Read the model definition and answer for the solid it produces. Units are mm, in the model's axes. Face numbers are marked on the shaded views. A direction names the side the tool comes from. Coordinates: 2 decimals unless noted, no trailing zeros. Write each loop counter-clockwise with the first axis right and the second up, starting at its lowest first coordinate (ties: lowest second). Pieces come first, ordered by that corner, then holes. Notation, with made-up numbers: (-12.5, -6) -> (22.5, -6) arc R17 ccw to (22.5, 20) -> close; hole circle Ø4 at (-33.75, 73.25). An arc over 180 degrees is marked (long way). One line per item, written item: value. Start each with the question number.
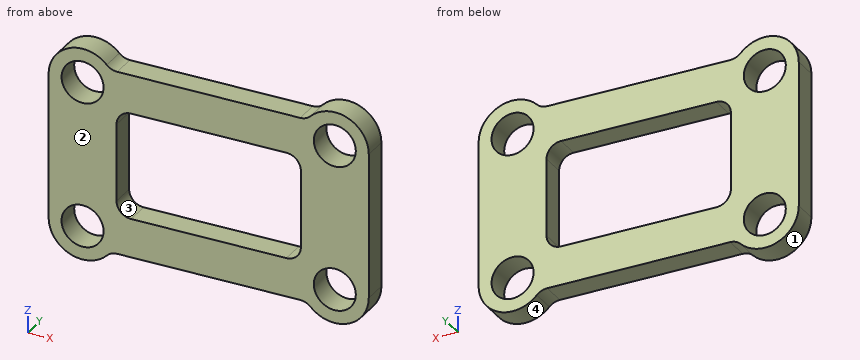
from build123d import *

# Parameters (mm, degrees)
BOSS_EXTRUDE2_DEPTH   = 3.175
BOSS_EXTRUDE2_2_DEPTH = 3.175
SKETCH7_W             = 33.02
SKETCH7_H             = 5.08
EXTRUDE_THIN1_DEPTH   = 3.175
M5_CLEARANCE_HOLE1_D  = 5.5
FILLET1_R             = 1.905


with BuildPart() as part:
    # Sketch1 → Boss-Extrude2 (new body)
    with BuildSketch(Plane.XZ.offset(19.05)):
        with BuildLine():
            Line((-24.765, 9.525), (-24.765, -9.525))
            ThreePointArc((-24.765, -9.525), (-29.21, -13.97), (-33.655, -9.525))
            Line((-33.655, -9.525), (-33.655, 9.525))
            ThreePointArc((-33.655, 9.525), (-29.21, 13.97), (-24.765, 9.525))
        make_face()
    extrude(amount=BOSS_EXTRUDE2_DEPTH)



with BuildPart() as body_2:
    # Sketch1 → Boss-Extrude2 2 (new body)
    with BuildSketch(Plane.XZ.offset(19.05)):
        with BuildLine():
            Line((8.255, 9.525), (8.255, -9.525))
            ThreePointArc((8.255, -9.525), (3.81, -13.97), (-0.635, -9.525))
            Line((-0.635, -9.525), (-0.635, 9.525))
            ThreePointArc((-0.635, 9.525), (3.81, 13.97), (8.255, 9.525))
        make_face()
    extrude(amount=BOSS_EXTRUDE2_2_DEPTH)


with BuildPart() as part_1:
    add(part.part)

    add(body_2.part)  # Extrude-Thin1 merges body 2
    # Sketch7 → Extrude-Thin1 (add)
    with BuildSketch(Plane.XZ.offset(22.225)):
        with Locations((-12.7, 9.525)):
            Rectangle(SKETCH7_W, SKETCH7_H)
        with Locations((-12.7, -9.525)):
            Rectangle(SKETCH7_W, SKETCH7_H)
    extrude(amount=-EXTRUDE_THIN1_DEPTH)

    # M5 Clearance Hole1 (through all)
    with Locations(Plane(origin=(-29.21, -22.225, 9.525), x_dir=(0, 0, -1), z_dir=(0, -1, 0))):
        with Locations((0, 0), (19.05, 0), (0, 33.02), (19.05, 33.02)):
            Hole(M5_CLEARANCE_HOLE1_D / 2)

    # Fillet1
    fillet1_edges = [part_1.edges().sort_by_distance(p)[0] for p in [
        (-25.562202719, -20.6375, 12.065),
        (-24.765, -20.6375, 6.985),
        (-0.635, -20.6375, 6.985),
        (0.162202719, -20.6375, 12.065),
        (0.162202719, -20.6375, -12.065),
        (-0.635, -20.6375, -6.985),
        (-24.765, -20.6375, -6.985),
        (-25.562202719, -20.6375, -12.065),
    ]]
    fillet(fillet1_edges, radius=FILLET1_R)


solid = part_1.part
1. A cutting plane is placed at D-D on x = -3. Give the vertices of the cut face in (y, z) (3 decimals).
2. A cutting plane is placed at A-A on y = -20.95. Count the separate pieces of the cut face and the enclosed holes in it, then the cut area to 3 significant figures.
3. A cutting plane is placed at C-C on z = -0.5. Give the vertices of the cut face in (x, y) (3 decimals).
4. Find the intervals of material crossed by probe 1 along Z at (x, y) = (-2.5, -20.95) (3 decimals); probe 2 along X at (y, z) = (-20.35, -8) (3 decimals); probe 3 along X at (y, z) = (-20.05, -11.75), in increasing order. Write a range as from..to.
5. A tool of negligible diameter and unlimited length cuts with its end or side. For the marked faces 3 and 4, from which of +Z, -Z, +X, -X, +Y, -Y can it reach the whole face along a straight path? Write none if from no direction.
6. Given pin 1 (4.5 mm diameter, centred on x = -29.21, z = -9.525, fed in from +Y); pin 2 (1.6 mm diameter, centred on x = -14, y = -20.5, fed in from +Z) (3 decimals); pin 3 (1 mm diameter, centred on x = -12.5, y = -21, fed in from -Z) (3 decimals), each flat-ended and moving along its own axis, determine where each tip first touches the part or whether it passes through.
7. A cutting plane is placed at B-B on x = 3.81. Give the vertices of the cut face in (y, z) (3 decimals).
8. For a pull along X with two mould halves and no side action, classify the marked faces 1 and 2 as +X half, -X half, draft (parallel to the pull), parting line (faces both ways), or undercut.
Derived:
1. outline: (-22.225, -12.065) -> (-19.05, -12.065) -> (-19.05, -6.985) -> (-22.225, -6.985) -> close; (-22.225, 6.985) -> (-19.05, 6.985) -> (-19.05, 12.065) -> (-22.225, 12.065) -> close
2. separate pieces: 1
2. enclosed holes: 5
2. area: 619 mm2
3. outline: (-33.655, -22.225) -> (-24.765, -22.225) -> (-24.765, -19.05) -> (-33.655, -19.05) -> close; (-0.635, -22.225) -> (8.255, -22.225) -> (8.255, -19.05) -> (-0.635, -19.05) -> close
4. probe 1: z = -12.065..-6.985, 6.985..12.065
4. probe 2: x = -33.655..-31.498, -26.922..1.522, 6.098..8.255
4. probe 3: x = -33.06..-30.83, -27.59..2.19, 5.43..7.66
5. face 3: +Y, -Y
5. face 4: -Z, +Y, -Y
6. pin 1: passes through
6. pin 2: stops at z = 12.065
6. pin 3: stops at z = -12.065
7. outline: (-22.225, -13.97) -> (-19.05, -13.97) -> (-19.05, -12.275) -> (-22.225, -12.275) -> close; (-22.225, -6.775) -> (-19.05, -6.775) -> (-19.05, 6.775) -> (-22.225, 6.775) -> close; (-22.225, 12.275) -> (-19.05, 12.275) -> (-19.05, 13.97) -> (-22.225, 13.97) -> close
8. face 1: undercut
8. face 2: draft
